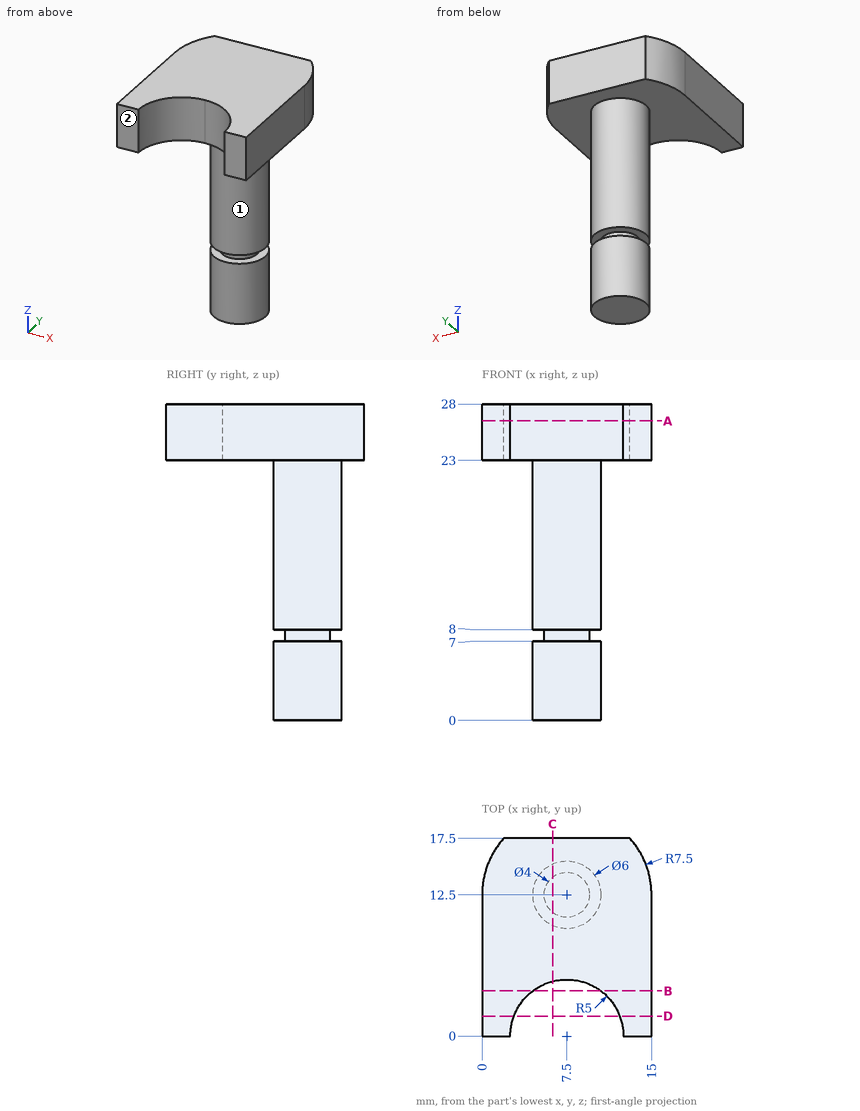
Part print with two shaded views. Sizes in mm from the minimum x, y, z corner. A direction names the side the tool comes from. Round coordinates to 2 decimals unless told otherwise and drop trailing zeros. Loops run counter-clockwise (first coordinate to the right, second up) from the corner with the lowest first, then second, coordinate; pieces in that order, holes last. Notation, with made-up numbers: M -34.5,-26 L 17.5,-26 A23 cw 17.5,7 Z; hole C 67.5,40.25 d1. An arc over 180 degrees is marked long. Put each result on its own line as item: value. Start each with the question number.
Item 1: Drop flat-ended pins along their axis: P1, Ø3, axis at x = 7, z = 9, coming from the +Y side; P2, Ø5, axis at y = 7.5, z = 13.5, coming from the +X side. Give the stop position or say it passes through.
Item 2: Cut at D-D (y = 1.75). List the corners of the cut face in (x, z), then the cut area to 3 significant figures.
Item 3: Cut at B-B (y = 4). List the corners of the cut face in (x, z), then the cut area to 3 significant figures.
Item 4: Cut at A-A (z = 26.5). List the corners of the cut face in (x, y).
Item 5: Cut at C-C (x = 6.25). List the corners of the cut face in (y, z).
Item 6: 3-axis set-ups, long thin cutter, end or side, ignore diameter. For the marked faces 1 and 2: which of +Z, -Z, +X, -X, +Y, -Y reach the whole face in a straight line?
Item 7: Drill centre lines: line 1 along Z through (x, y) = (5.25, 13.5); line 2 along Z through (x, y) = (12.75, 14.25); line 3 along X through (y, z) = (1.75, 25). Where is each one in solid material? Low to high.
Answer block:
1. P1: y = 15.5
1. P2: x = 9.16
2. outline: M 0,23 L 2.82,23 L 2.82,28 L 0,28 Z; M 12.18,23 L 15,23 L 15,28 L 12.18,28 Z
2. area: 28.2 mm2
3. outline: M 0,23 L 4.5,23 L 4.5,28 L 0,28 Z; M 10.5,23 L 15,23 L 15,28 L 10.5,28 Z
3. area: 45.0 mm2
4. outline: M 0,0 L 2.5,0 A5 cw 12.5,0 L 15,0 L 15,12.5 A7.5 ccw 13.09,17.5 L 1.91,17.5 A7.5 ccw 0,12.5 Z
5. outline: M 4.84,23 L 9.77,23 L 9.77,8 L 10.94,8 L 10.94,7 L 9.77,7 L 9.77,0 L 15.23,0 L 15.23,7 L 14.06,7 L 14.06,8 L 15.23,8 L 15.23,23 L 17.5,23 L 17.5,28 L 4.84,28 Z
6. face 1: -Z
6. face 2: +Z, -Z, +X, -X, -Y
7. line 1: 0 to 7, 8 to 28
7. line 2: 23 to 28
7. line 3: 0 to 2.82, 12.18 to 15
